Input: part model. Units: mm. Frame: model coordinates. A direction names the side the tool comes from. Coordinates: 2 decimals unless noted, no trailing zeros. Order: outer loops, then holes, each group sorted by start corner. A loop starts at its lowest first (then second) coordinate and runs counter-clockwise, first axis right, second up. Notation, with made-up numbers: M 31.25,68 L 82.25,68 A25 ccw 82.25,107 Z; hole C 82,37.5 d6. An arc over 180 degrees is marked long. One line per item, written item: value.
```python
from build123d import *

# Parameters (mm, degrees)
F1_DEPTH = 3


with BuildPart() as f1:
    # F0 (on Top) → F1 (new body)
    with BuildSketch(Plane.XY):
        Polygon((-92.604274, -0.498616), (-92.604274, -120.498616), (-42.604274, -120.498616), (-42.604274, -0.498616), (-39.604274, -0.498616), (-39.604274, 19.501384), (-42.604274, 19.501384), (-92.604274, 19.501384), (-95.604274, 19.501384), (-95.604274, -0.498616), align=None)
        with BuildLine():
            Line((-69.104274, -115.498616), (-69.104274, -45.498616))
            ThreePointArc((-69.104274, -45.498616), (-67.604274, -43.998616), (-66.104274, -45.498616))
            Line((-66.104274, -45.498616), (-66.104274, -115.498616))
            ThreePointArc((-66.104274, -115.498616), (-67.604274, -116.998616), (-69.104274, -115.498616))
        make_face(mode=Mode.SUBTRACT)
    extrude(amount=F1_DEPTH)


solid = f1.part
```
(1) Draft query along X for faces 5 (the flat face through (-42.604, -61, 1)), 6 (the flat face through (-95.604, 10, 1)), 7 (the cylindrical face through (-67.6, -44, 1.5)). Return one class per face: released by +X, released by -X, zero draft, split by the parting line, or undercut.
Data:
face 5: released by +X
face 6: released by -X
face 7: undercut
(2) Cut plane B-B on z = 0.6. Output: boundary loops of the cut face in (x, y).
Data:
outline: M -95.6,-0.5 L -92.6,-0.5 L -92.6,-120.5 L -42.6,-120.5 L -42.6,-0.5 L -39.6,-0.5 L -39.6,19.5 L -95.6,19.5 Z; hole M -69.1,-115.5 A1.5 ccw -66.1,-115.5 L -66.1,-45.5 A1.5 ccw -69.1,-45.5 Z
(3) First-contact query: pin 1 (0.9 mm diameter, centred on y = -91, z = 2, fed in from +X); pin 2 (0.9 mm diameter, centred on x = -93.5, z = 1, fed in from -Y). Flat tips, straight axial feed; report the tip coordinate or a pass-through.
Data:
pin 1: stops at x = -42.6
pin 2: stops at y = -0.5
(4) Cut plane C-C on y = -24.5. Output: boundary loops of the cut face in (x, z).
Data:
outline: M -92.6,0 L -42.6,0 L -42.6,3 L -92.6,3 Z
(5) Cut plane A-A on y = -89. Output: boundary loops of the cut face in (x, z).
Data:
outline: M -92.6,0 L -69.1,0 L -69.1,3 L -92.6,3 Z; M -66.1,0 L -42.6,0 L -42.6,3 L -66.1,3 Z
(6) Access query for faces 1 (the flat face through (-66.104, -80, 1)), 2 (the flat face through (-92.604, -60, 1)), 3 (the flat face through (-62, -50, 0)), 4 (the flat face through (-41, -0.499, 1)). Directions: +Z, -Z, +X, -X, +Y, -Y. A direction counts if a zero-diameter tool reaches every point of the face in a straight line with its end or side. Return the directions, or none.
Data:
face 1: +Z, -Z
face 2: +Z, -Z, -X, -Y
face 3: -Z, +X, -X, +Y, -Y
face 4: +Z, -Z, +X, -Y
(7) Ray query, line 1 (X direction, y = -63.5, z = 1.8); line 2 (X direction, y = -19, z = 1.15). Return the intervals inside material, ascending. Write a range as from..to.
Data:
line 1: x = -92.6..-69.1, -66.1..-42.6
line 2: x = -92.6..-42.6
